from build123d import *

# Parameters (mm, degrees)
ESBO_O1_R                = 11
ESBO_O1_R_2              = 1.6
RESSALTO_EXTRUS_O1_DEPTH = 3
FILETE1_R                = 5


with BuildPart() as part:
    # Esboço1 → Ressalto-extrusão1 (new body)
    with BuildSketch(Plane.XY):
        with BuildLine():
            Line((-15.491933385, -4), (-29, -4))
            Line((-29, -4), (-6.831996166, -14.468027799))
            ThreePointArc((-6.831996166, -14.468027799), (-12.328193669, -10.198805854), (-15.491933385, -4))
        make_face()
        with BuildLine():
            Line((-29, -4), (-15.491933385, -4))
            ThreePointArc((-15.491933385, -4), (0, -16), (15.491933385, -4))
            Line((15.491933385, -4), (29, -4))
            Line((29, -4), (29, 4))
            Line((29, 4), (15.491933385, 4))
            ThreePointArc((15.491933385, 4), (0, 16), (-15.491933385, 4))
            Line((-15.491933385, 4), (-29, 4))
            Line((-29, 4), (-29, -4))
        make_face()
        Circle(ESBO_O1_R, mode=Mode.SUBTRACT)
        with Locations((-25, 0)):
            Circle(ESBO_O1_R_2, mode=Mode.SUBTRACT)
        with Locations((25, 0)):
            Circle(ESBO_O1_R_2, mode=Mode.SUBTRACT)
        with BuildLine():
            Line((-6.831996166, 14.468027799), (-29, 4))
            Line((-29, 4), (-15.491933385, 4))
            ThreePointArc((-15.491933385, 4), (-12.328193669, 10.198805854), (-6.831996166, 14.468027799))
        make_face()
        with BuildLine():
            ThreePointArc((15.491933385, -4), (12.328193669, -10.198805854), (6.831996166, -14.468027799))
            Line((6.831996166, -14.468027799), (29, -4))
            Line((29, -4), (15.491933385, -4))
        make_face()
        with BuildLine():
            Line((29, 4), (6.831996166, 14.468027799))
            ThreePointArc((6.831996166, 14.468027799), (12.328193669, 10.198805854), (15.491933385, 4))
            Line((15.491933385, 4), (29, 4))
        make_face()
    extrude(amount=RESSALTO_EXTRUS_O1_DEPTH)

    # Filete1
    filete1_edges = [part.edges().sort_by_distance(p)[0] for p in [
        (29, 4, 1.5),
        (29, -4, 1.5),
        (-29, -4, 1.5),
        (-29, 4, 1.5),
    ]]
    fillet(filete1_edges, radius=FILETE1_R)


solid = part.part
Work out the finished part from the listing and answer in its coordinate system (mm). Give positions to 0.01 mm unless a question says otherwise; leave off trailing zeros. Order: outer loops, then holes, each group sorted by start corner. A loop starts at its lowest first (then second) coordinate and runs counter-clockwise, first axis right, second up. Notation, with made-up numbers: (-14.75, 33) -> (2.25, 33) arc R20 ccw to (2.25, 64) -> close; hole circle Ø7 at (-0.5, 49.5). An arc over 180 degrees is marked (long way). Answer as a JSON object with one key per item and string values. Group by question number.
1. Section A-A on z = 1.65 is taken. Determine the outline of the cut face in (x, y) (3 decimals).
2. Section C-C on x = 10 is taken. Determine the outline of the cut face in (y, z).
3. Consider line 1 along X through (y, z) = (-2.5, 0.15); line 2 along Y through (x, z) = (-1, 2.6); line 3 along Y through (x, z) = (5, 1.9). Determine where each line is inside the solid, lowest interval first. Write a range as [from, to].
4. Section D-D on x = 18 is taken. Determine the outline of the cut face in (y, z), plus the area to 3 significant figures.
5. The mould has two halves that part along Y. Classify faces 1 (the cylindrical face through (-26.18, 1.08, 1.48)), 2 (the flat face through (-16.619, -9.847, 1.479)), 3 (the flat face through (-7, 11, 3)), 4 (the cylindrical face through (23.82, 1.08, 1.48)): released by +Y, released by -Y, zero draft, split by the parting line, or undercut.
6. A flat-ended cylindrical pin translates along its axis: pin 1 Ø1.5 at (x, z) = (13, 2.5) entering from +Y. Find the tip coordinate at first contact, or state that the pin passes through.
7. Section B-B on x = 0 is taken. Determine the outline of the cut face in (y, z), plus the area to 3 significant figures.
Result sheet:
{
 "1": {"outline": "(-29, -0.832) arc R5 ccw to (-26.135, -5.353) -> (-6.832, -14.468) arc R16 ccw to (6.832, -14.468) -> (26.135, -5.353) arc R5 ccw to (29, -0.832) -> (29, 0.832) arc R5 ccw to (26.135, 5.353) -> (6.832, 14.468) arc R16 ccw to (-6.832, 14.468) -> (-26.135, 5.353) arc R5 ccw to (-29, 0.832) -> close; hole circle Ø3.2 at (-25, 0); hole circle Ø22 at (0, 0); hole circle Ø3.2 at (25, 0)"},
 "2": {"outline": "(-12.97, 0) -> (-4.58, 0) -> (-4.58, 3) -> (-12.97, 3) -> close; (4.58, 0) -> (12.97, 0) -> (12.97, 3) -> (4.58, 3) -> close"},
 "3": {"line 1": "x = [-28.71, -10.71], [10.71, 28.71]", "line 2": "y = [-15.97, -10.95], [10.95, 15.97]", "line 3": "y = [-15.2, -9.8], [9.8, 15.2]"},
 "4": {"outline": "(-9.19, 0) -> (9.19, 0) -> (9.19, 3) -> (-9.19, 3) -> close", "area": "55.2 mm^2"},
 "5": {"face 1": "undercut", "face 2": "released by -Y", "face 3": "zero draft", "face 4": "undercut"},
 "6": {"pin 1": "stops at y = 11.91"},
 "7": {"outline": "(-16, 0) -> (-11, 0) -> (-11, 3) -> (-16, 3) -> close; (11, 0) -> (16, 0) -> (16, 3) -> (11, 3) -> close", "area": "30.0 mm^2"}
}
